CAD build for the part. Positions are in the model's coordinates, mm. A direction names the side the tool comes from. Coordinates: 2 decimals unless noted, no trailing zeros. Loops run counter-clockwise (first coordinate to the right, second up) from the corner with the lowest first, then second, coordinate; pieces in that order, holes last. Notation, with made-up numbers: (48, 11.5) -> (90, 11.5) arc R10 cw to (90, 16.5) -> close; hole circle Ø8 at (-26.5, -4). An arc over 180 degrees is marked (long way). Answer as CSV lines item,"result". Start each with the question number.
from build123d import *

# Parameters (mm, degrees)
BOSS_EXTRUDE1_DEPTH = 15
CUT_EXTRUDE1_REACH  = 32.773
SKETCH2_R           = 1.525
SKETCH3_R           = 2.75
CUT_EXTRUDE2_DEPTH  = 3
CUT_EXTRUDE3_REACH  = 32.773
SKETCH4_R           = 0.4


with BuildPart() as part:
    # Sketch1 → Boss-Extrude1 (new body)
    with BuildSketch(Plane(origin=(0, 0, 0), x_dir=(1, 0, 0), z_dir=(0, 1, 0))):
        with BuildLine():
            Line((1, 0), (18, 0))
            ThreePointArc((18, 0), (18.707106781, 0.292893219), (19, 1))
            Line((19, 1), (19, 18))
            ThreePointArc((19, 18), (18.707106781, 18.707106781), (18, 19))
            Line((18, 19), (1, 19))
            ThreePointArc((1, 19), (0.292893219, 18.707106781), (0, 18))
            Line((0, 18), (0, 1))
            ThreePointArc((0, 1), (0.292893219, 0.292893219), (1, 0))
        make_face()
    extrude(amount=BOSS_EXTRUDE1_DEPTH)

    # Sketch2 → Cut-Extrude1 (cut, up to next)
    with BuildSketch(Plane(origin=(0, 15, 0), x_dir=(1, 0, 0), z_dir=(0, 1, 0)), mode=Mode.PRIVATE) as cut_extrude1_sk1:
        with Locations(Location((3.25, 9.5, 0), (0, 0, 270))):
            Circle(SKETCH2_R)
    cut_extrude1_tool1 = extrude(cut_extrude1_sk1.sketch, amount=-CUT_EXTRUDE1_REACH, mode=Mode.PRIVATE) & part.part
    # Sketch2 → Cut-Extrude1 (cut, up to next)
    with BuildSketch(Plane(origin=(0, 15, 0), x_dir=(1, 0, 0), z_dir=(0, 1, 0)), mode=Mode.PRIVATE) as cut_extrude1_sk2:
        with Locations(Location((15.75, 9.5, 0), (0, 0, 270))):
            Circle(SKETCH2_R)
    cut_extrude1_tool2 = extrude(cut_extrude1_sk2.sketch, amount=-CUT_EXTRUDE1_REACH, mode=Mode.PRIVATE) & part.part
    add(cut_extrude1_tool1.solids().sort_by_distance((3.25, 15, -9.5))[0], mode=Mode.SUBTRACT)
    add(cut_extrude1_tool2.solids().sort_by_distance((15.75, 15, -9.5))[0], mode=Mode.SUBTRACT)

    # Sketch3 → Cut-Extrude2 (cut)
    with BuildSketch(Plane(origin=(0, 15, 0), x_dir=(1, 0, 0), z_dir=(0, 1, 0))):
        with Locations(Location((3.25, 9.5, 0), (0, 0, 270))):
            Circle(SKETCH3_R)
        with Locations(Location((15.75, 9.5, 0), (0, 0, 270))):
            Circle(SKETCH3_R)
    extrude(amount=-CUT_EXTRUDE2_DEPTH, mode=Mode.SUBTRACT)

    # Sketch4 → Cut-Extrude3 (cut, up to next)
    with BuildSketch(Plane.ZY, mode=Mode.PRIVATE) as cut_extrude3_sk1:
        with Locations((-16.458209363, 13.587683821)):
            Circle(SKETCH4_R)
    cut_extrude3_tool1 = extrude(cut_extrude3_sk1.sketch, amount=-CUT_EXTRUDE3_REACH, mode=Mode.PRIVATE) & part.part
    add(cut_extrude3_tool1.solids().sort_by_distance((0, 13.587684, -16.458209))[0], mode=Mode.SUBTRACT)


solid = part.part
Item 1: Saw through at B-B (y = 8.5). Write the cut outline in (x, z) (3 decimals).
Item 2: Saw through at A-A (z = -9.5). Write the cut outline in (x, y) (3 decimals), plus the area to 3 significant figures.
Item 3: Wall check: probe 1 along X at (y, z) = (13.25, -9.5); probe 2 along X at (y, z) = (3.25, -10.5); probe 3 along Z at (x, y) = (14.25, 13.75). Give the ranges that are in metal, low to high.
Item 4: Which spindle directions (+Z, -Z, +X, -X, +Y, -Y) get a long thin tool onto all of the face, cutting with end or side? Do faces 4 (the face through (0.285, 7.395, -0.301)), 5 (the face through (2.2, 13.52, -6.96)). Say none if no direction does.
Item 5: Two-plate mould, pull along Z, no slides. Class faces 1 (the face through (19, 7, -9)), 2 (the face through (18.715, 7.395, -18.699)), 3 (the face through (15, 12, -8)): pulls with the +Z half, pulls with the -Z half, needs draft (parallel to the pull), parting line crosses it, or undercut.
Item 6: Saw through at C-C (x = 3.25). Write the cut outline in (y, z) (3 decimals).
Item 7: Flat gauge pins, fed straight in: pin 1 Ø1.8 at (x, z) = (15.75, -9.5) entering from -Y; pin 2 Ø4 at (x, z) = (3.25, -9.5) entering from +Y. Where does each tip first touch, or does it go through?
Geometry check:
1,outline,"(0, -18) arc R1 ccw to (1, -19) -> (18, -19) arc R1 ccw to (19, -18) -> (19, -1) arc R1 ccw to (18, 0) -> (1, 0) arc R1 ccw to (0, -1) -> close; hole circle Ø3.05 at (3.25, -9.5); hole circle Ø3.05 at (15.75, -9.5)"
2,outline,"(0, 0) -> (1.725, 0) -> (1.725, 12) -> (0.5, 12) -> (0.5, 15) -> (0, 15) -> close; (4.775, 0) -> (14.225, 0) -> (14.225, 12) -> (13, 12) -> (13, 15) -> (6, 15) -> (6, 12) -> (4.775, 12) -> close; (17.275, 0) -> (19, 0) -> (19, 15) -> (18.5, 15) -> (18.5, 12) -> (17.275, 12) -> close"
2,area,"179 mm2"
3,probe 1,"0 to 0.5, 6 to 13, 18.5 to 19"
3,probe 2,"0 to 2.1, 4.4 to 14.6, 16.9 to 19"
3,probe 3,"-19 to -16.82, -16.09 to -11.8, -7.2 to 0"
4,face 4,"+Z, -X, +Y, -Y"
4,face 5,"+Y"
5,face 1,"needs draft"
5,face 2,"pulls with the -Z half"
5,face 3,"undercut"
6,outline,"(0, -19) -> (15, -19) -> (15, -12.25) -> (12, -12.25) -> (12, -11.025) -> (0, -11.025) -> close; (0, -7.975) -> (12, -7.975) -> (12, -6.75) -> (15, -6.75) -> (15, 0) -> (0, 0) -> close; hole circle Ø0.8 at (13.588, -16.458)"
7,pin 1,"through"
7,pin 2,"y = 12"
